Check sheet for the drawn part. Datum: minimum x, y, z corner. Units: mm. A direction names the side the tool comes from. Give positions to 0.01 mm unless a question says otherwise; leave off trailing zeros. Write each loop counter-clockwise with the first axis right and the second up, starting at its lowest first coordinate (ties: lowest second). Pieces come first, ordered by that corner, then holes. Notation, with made-up numbers: (73.25, -39) - (83.25, -39) arc R25 cw to (83.25, -6) - close; hole circle Ø3 at (-27.75, 88.25). An arc over 180 degrees is marked (long way). One line per question, with ' | ' between items. Start each with the question number.
Q1. Thickness scan on L1, parallel to X at y = 35.5, z = 5.08; L2, parallel to Y at x = 5.75, z = 15.5; L3, parallel to Y at x = 14.75, z = 28. Record the ranges inside material, lowest first. Write a range as [from, to].
Q2. Gauge pin test, flat ends, axial feed: P1, Ø1.5, axis at x = 10.5, y = 9.5, coming from the -Z side; P2, Ø1.4, axis at x = 3.57, y = 28.18, coming from the -Z side. Record the tip position at first contact, or that the pin passes through.
Q3. Section check C-C on x = 16.5. Record the boundary of the cut face in (y, z).
Q4. Section check D-D on y = 25. Record the boundary of the cut face in (x, z), and give its area (3 significant figures).
Q5. Set-up check for the marked faces 4 and 5: record each of +Z, -Z, +X, -X, +Y, -Y from which the full face is reachable in a straight line by a thin tool's end or side.
Q6. Section check A-A on z = 20.32. Record the boundary of the cut face in (x, y).
Q7. Release check for a two-part mould opening along Y. For the marked faces 1, 2 and 3 record: +Y half, -Y half, draft (parallel to the pull), parting line (faces both ways), or undercut.
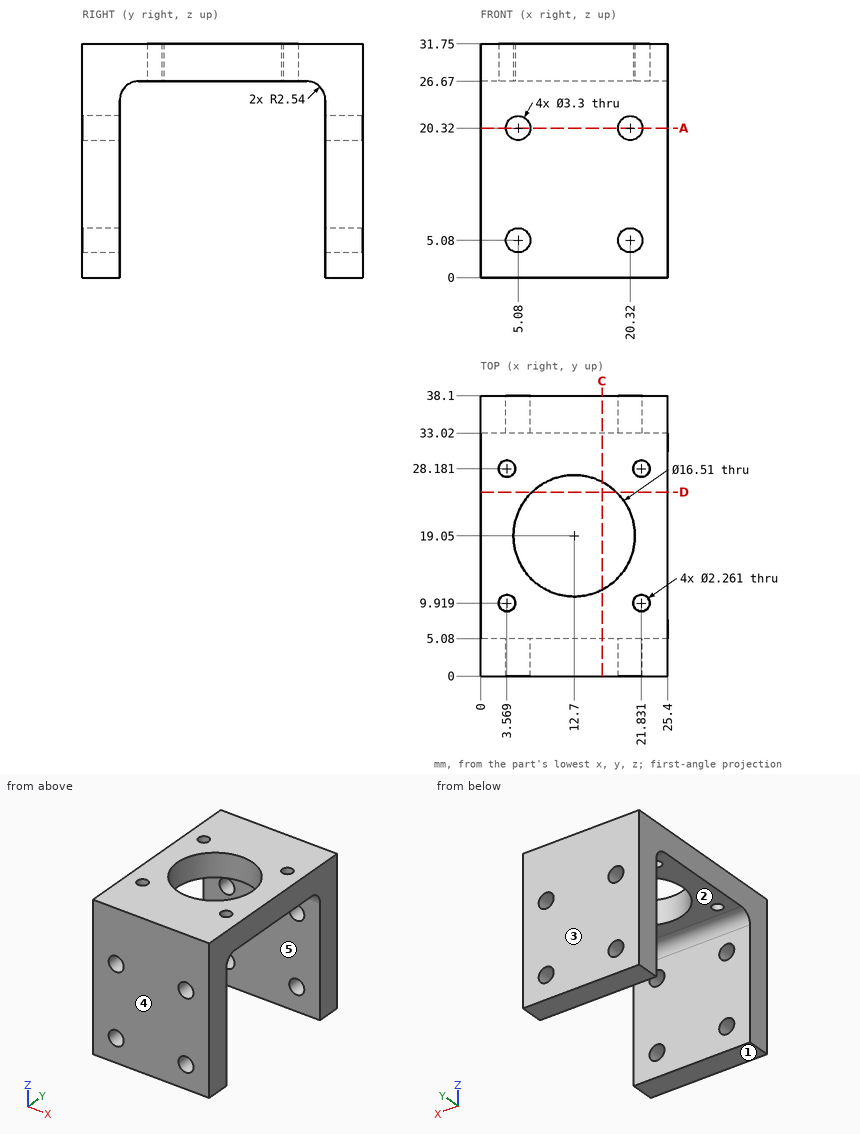
Working result:
1) L1: x = [0, 3.43], [6.73, 18.67], [21.97, 25.4] | L2: y = [0, 5.08], [33.02, 38.1] | L3: y = [0, 11.05], [27.05, 38.1]
2) P1: stops at z = 26.67 | P2: passes through
3) outline: (0, 0) - (5.08, 0) - (5.08, 24.13) arc R2.54 cw to (7.62, 26.67) - (11.72, 26.67) - (11.72, 31.75) - (0, 31.75) - close; (26.38, 26.67) - (30.48, 26.67) arc R2.54 cw to (33.02, 24.13) - (33.02, 0) - (38.1, 0) - (38.1, 31.75) - (26.38, 31.75) - close
4) outline: (0, 26.67) - (6.98, 26.67) - (6.98, 31.75) - (0, 31.75) - close; (18.42, 26.67) - (25.4, 26.67) - (25.4, 31.75) - (18.42, 31.75) - close | area: 70.9 mm2
5) face 4: +Z, -Z, +X, -X, -Y | face 5: -Z, +X, -X
6) outline: (0, 0) - (3.43, 0) - (3.43, 5.08) - (0, 5.08) - close; (0, 33.02) - (3.43, 33.02) - (3.43, 38.1) - (0, 38.1) - close; (6.73, 0) - (18.67, 0) - (18.67, 5.08) - (6.73, 5.08) - close; (6.73, 33.02) - (18.67, 33.02) - (18.67, 38.1) - (6.73, 38.1) - close; (21.97, 0) - (25.4, 0) - (25.4, 5.08) - (21.97, 5.08) - close; (21.97, 33.02) - (25.4, 33.02) - (25.4, 38.1) - (21.97, 38.1) - close
7) face 1: draft | face 2: undercut | face 3: +Y half
